For this review, take the finished solid that the model builds, in its own axes (mm). Face numbers are marked on the shaded views. A direction names the side the tool comes from. Round coordinates to 2 decimals unless told otherwise and drop trailing zeros. Loops run counter-clockwise (first coordinate to the right, second up) from the corner with the lowest first, then second, coordinate; pieces in that order, holes last.
1. Draft analysis for pull direction Y (two halves, no side actions). For the marked faces 3, 4 and 5, state which applies: released by +Y, released by -Y, zero draft, split by the parting line, or undercut.
2. Consider section A-A on z = 0. State the section outline as (x, y) points.
3. To check wall thickness, follow line 1 along Z through (x, y) = (3.7, 0); line 2 along Z through (x, y) = (1.9, 0); line 3 along X through (y, z) = (5.5, 6.5). State the ranges of each line that lie inside material, in increasing order.
4. Consider section D-D on y = 7.5. State the section outline as (x, z) points, then the cut area to 3 significant figures.
5. Tool access review of the marked faces 1 and 2: name each direction out of +Z, -Z, +X, -X, +Y, -Y from which nothing blocks a thin tool from reaching the whole face with its end or side.
6. Consider section C-C on z = 8.5. State the section outline as (x, y) points.
7. Clearance check with flat-ended pins moving along their axes: pin 1 Ø1.5 at (y, z) = (6, 5) entering from -X; pin 2 Ø1 at (x, y) = (2, 1.5) entering from -Z; pin 3 Ø1.5 at (x, z) = (1, -2) entering from -Y. State where each tip first meets the part, or that it passes through.
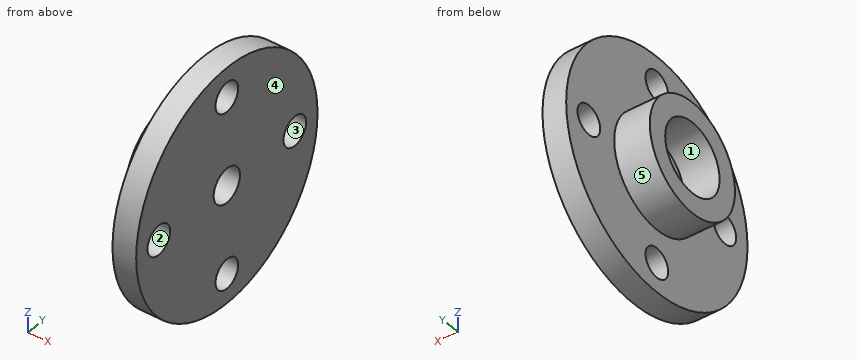
from build123d import *

# Parameters (mm, degrees)
ESQUISSE2_R             = 1.45
ESQUISSE2_R_2           = 1.25
ENL_V_MAT_EXTRU_1_DEPTH = 10


with BuildPart() as part:
    # Esquisse1 → Révolution1 (revolve)
    with BuildSketch(Plane.XY):
        Polygon((0, 3), (0, 4.7), (3, 4.7), (3, 10), (5, 10), (5, 0), (3, 0), (3, 3), align=None)
    revolve(axis=Axis((5, 0, 0), (-1, 0, 0)))

    # Esquisse2 → Enlèv. mat.-Extru.1 (cut)
    with BuildSketch(Plane(origin=(5, 0, 0), x_dir=(0, 0, -1), z_dir=(1, 0, 0))):
        with Locations(Location((0, 0, 0), (0, 0, 90))):
            Circle(ESQUISSE2_R)
        with Locations(Location((0, 7.5, 0), (0, 0, 90))):
            Circle(ESQUISSE2_R_2)
        with Locations(Location((7.5, 0, 0), (0, 0, 90))):
            Circle(ESQUISSE2_R_2)
        with Locations(Location((0, -7.5, 0), (0, 0, 90))):
            Circle(ESQUISSE2_R_2)
        with Locations(Location((-7.5, 0, 0), (0, 0, 90))):
            Circle(ESQUISSE2_R_2)
    extrude(amount=-ENL_V_MAT_EXTRU_1_DEPTH, mode=Mode.SUBTRACT)


solid = part.part
Resolved:
1. face 3: undercut
1. face 4: zero draft
1. face 5: split by the parting line
2. outline: (0, -4.7) - (3, -4.7) - (3, -6.25) - (5, -6.25) - (5, -1.45) - (3, -1.45) - (3, -3) - (0, -3) - close; (0, 3) - (3, 3) - (3, 1.45) - (5, 1.45) - (5, 6.25) - (3, 6.25) - (3, 4.7) - (0, 4.7) - close; (3, -10) - (5, -10) - (5, -8.75) - (3, -8.75) - close; (3, 8.75) - (5, 8.75) - (5, 10) - (3, 10) - close
3. line 1: z = -10 to -8.75, -6.25 to -1.45, 1.45 to 6.25, 8.75 to 10
3. line 2: z = -4.7 to -3, 3 to 4.7
3. line 3: x = 3 to 5
4. outline: (3, -6.61) - (5, -6.61) - (5, -1.25) - (3, -1.25) - close; (3, 1.25) - (5, 1.25) - (5, 6.61) - (3, 6.61) - close
4. area: 21.5 mm2
5. face 1: -X
5. face 2: +X, -X
6. outline: (3, -5.27) - (5, -5.27) - (5, -0.75) - (3, -0.75) - close; (3, 0.75) - (5, 0.75) - (5, 5.27) - (3, 5.27) - close
7. pin 1: stops at x = 3
7. pin 2: stops at z = -4.59
7. pin 3: stops at y = -4.53
